from build123d import *

# Parameters (mm, degrees)
SKETCH1_R           = 4
BOSS_EXTRUDE1_DEPTH = 19
SKETCH2_R           = 2.25
CUT_EXTRUDE2_DEPTH  = 19
SKETCH3_R           = 7
SKETCH3_R_2         = 4
BOSS_EXTRUDE2_DEPTH = 3
FILLET1_R           = 1


with BuildPart() as part:
    # Sketch1 → Boss-Extrude1 (new body)
    with BuildSketch(Plane.XY):
        with BuildLine():
            Line((-28.2, 0), (28.2, 0))
            Line((28.2, 0), (28.2, 6))
            Line((28.2, 6), (11.5, 6))
            ThreePointArc((11.5, 6), (10.085786438, 6.585786438), (9.5, 8))
            Line((9.5, 8), (9.5, 11.1))
            ThreePointArc((9.5, 11.1), (0, 20.6), (-9.5, 11.1))
            Line((-9.5, 11.1), (-9.5, 8))
            ThreePointArc((-9.5, 8), (-10.085786438, 6.585786438), (-11.5, 6))
            Line((-11.5, 6), (-28.2, 6))
            Line((-28.2, 6), (-28.2, 0))
        make_face()
        with Locations((0, 11.1)):
            Circle(SKETCH1_R, mode=Mode.SUBTRACT)
    extrude(amount=BOSS_EXTRUDE1_DEPTH)

    # Sketch2 → Cut-Extrude2 (cut)
    with BuildSketch(Plane.XZ):
        with BuildLine():
            Line((28.2, 19), (18.7, 19))
            ThreePointArc((18.7, 19), (25.417514421, 16.217514421), (28.2, 9.5))
            Line((28.2, 9.5), (28.2, 19))
        make_face()
        with BuildLine():
            ThreePointArc((-28.2, 9.5), (-25.417514421, 16.217514421), (-18.7, 19))
            Line((-18.7, 19), (-28.2, 19))
            Line((-28.2, 19), (-28.2, 9.5))
        make_face()
        with BuildLine():
            Line((28.2, 0), (28.2, 9.5))
            ThreePointArc((28.2, 9.5), (25.417514421, 2.782485579), (18.7, 0))
            Line((18.7, 0), (28.2, 0))
        make_face()
        with BuildLine():
            ThreePointArc((-18.7, 0), (-25.417514421, 2.782485579), (-28.2, 9.5))
            Line((-28.2, 9.5), (-28.2, 0))
            Line((-28.2, 0), (-18.7, 0))
        make_face()
        with Locations(Location((19, 9.5, 0), (0, 0, 270))):
            Circle(SKETCH2_R)
        with Locations(Location((-19, 9.5, 0), (0, 0, 270))):
            Circle(SKETCH2_R)
    extrude(amount=-CUT_EXTRUDE2_DEPTH, mode=Mode.SUBTRACT)

    # Sketch3 → Boss-Extrude2 (add)
    with BuildSketch(Plane.XY.offset(19)):
        with Locations((0, 11.1)):
            Circle(SKETCH3_R)
        with Locations((0, 11.1)):
            Circle(SKETCH3_R_2, mode=Mode.SUBTRACT)
    extrude(amount=BOSS_EXTRUDE2_DEPTH)

    # Fillet1
    fillet1_edges = [part.edges().sort_by_distance(p)[0] for p in [
        (10.085786438, 6.585786438, 19),
        (-15.1, 6, 0),
        (-10.085786438, 6.585786438, 0),
        (-9.5, 9.55, 0),
        (0, 20.6, 0),
        (9.5, 9.55, 0),
        (10.085786438, 6.585786438, 0),
        (9.5, 9.55, 19),
        (0, 20.6, 19),
        (-9.5, 9.55, 19),
        (-10.085786438, 6.585786438, 19),
        (-15.1, 6, 19),
        (0, 0, 19),
        (-28.2, 6, 9.5),
        (-28.2, 0, 9.5),
        (0, 0, 0),
        (15.1, 6, 19),
        (28.2, 0, 9.5),
        (28.2, 6, 9.5),
        (15.1, 6, 0),
    ]]
    fillet(fillet1_edges, radius=FILLET1_R)


solid = part.part
Design review of the part built by this model. Coordinates are the model's own, in mm. A direction names the side the tool comes from. Coordinates: 2 decimals unless noted, no trailing zeros. Loops run counter-clockwise (first coordinate to the right, second up) from the corner with the lowest first, then second, coordinate; pieces in that order, holes last.
Item 1: Add section B-B (x = -12.5). Write out the cut boundary in (y, z), and give its area (3 significant figures).
Completed:
outline: (0, 1) arc R1 ccw to (1, 0) - (5, 0) arc R1 ccw to (6, 1) - (6, 18) arc R1 ccw to (5, 19) - (1, 19) arc R1 ccw to (0, 18) - close
area: 113 mm2
Item 2: Draft analysis for pull direction Z (two halves, no side actions). For faces 6 (the cylindrical face through (16.804, 2.958, 9.988)), 7 (the cylindrical face through (-21.196, 2.958, 9.988)), 8 (the flat face through (0, 0, 9)), 9 (the cylindrical face through (15.05, 5.715, 18.699)), state which applies: pulls with the +Z half, pulls with the -Z half, needs draft (parallel to the pull), parting line crosses it, or undercut.
Completed:
face 6: undercut
face 7: undercut
face 8: needs draft
face 9: pulls with the +Z half
Item 3: Add section C-C (x = 17.5). Write out the cut boundary in (y, z), and give its area (3 significant figures).
Completed:
outline: (0, 1) arc R1 ccw to (1, 0) - (5, 0) arc R1 ccw to (6, 1) - (6, 7.82) - (0, 7.82) - close; (0, 11.18) - (6, 11.18) - (6, 18) arc R1 ccw to (5, 19) - (1, 19) arc R1 ccw to (0, 18) - close
area: 93.0 mm2
Item 4: Clearance check with flat-ended pins moving along their axes: pin 1 (6 mm diameter, centred on x = 12, y = 7, fed in from +Z); pin 2 (5 mm diameter, centred on x = -5.5, y = 15.5, fed in from +Z); pin 3 (8 mm diameter, centred on x = -20.5, z = 14.5, fed in from +Y); pin 4 (1.5 mm diameter, centred on y = 10, z = 7, fed in from +X). State where each tip first meets the part, or that it passes through.
Completed:
pin 1: stops at z = 19
pin 2: stops at z = 22
pin 3: stops at y = 6
pin 4: stops at x = 9.5
Item 5: For faces 1 (the cylindrical face through (-9.215, 9.528, 18.699)), 2 (the flat face through (9.5, 10, 9)), 3 (the cylindrical face through (-9.215, 9.572, 0.301)), 4 (the cylindrical face through (3.23, 4.89, 20.48)), 5 (the cylindrical face through (9.215, 9.572, 18.699)), list the 3-axis set-ups (+Z, -Z, +X, -X, +Y, -Y) from which the entire face can be reached by the end or side of a thin tool; tool diameter is ignored.
Completed:
face 1: +Z, -X, +Y
face 2: +Z, -Z, +X, +Y
face 3: -Z, -X, +Y
face 4: +Z
face 5: +Z, +X, +Y
Item 6: Add section A-A (y = 1.75). Write out the cut boundary in (x, z), and give its area (3 significant figures).
Completed:
outline: (-18.7, 0) - (18.7, 0) arc R9.5 ccw to (18.7, 19) - (-18.7, 19) arc R9.5 ccw to start; hole circle Ø4.5 at (-19, 9.5); hole circle Ø4.5 at (19, 9.5)
area: 962 mm2
Item 7: Wall thickness on L1, parallel to X at y = 2.65, z = 9.5; L2, parallel to X at y = 3, z = 11.5; L3, parallel to Y at x = 0, z = 11: over which ranges is each line inside the solid? List them lowest first.
Completed:
L1: x = -28.2 to -21.25, -16.75 to 16.75, 21.25 to 28.2
L2: x = -27.99 to -20.03, -17.97 to 17.97, 20.03 to 27.99
L3: y = 0 to 7.1, 15.1 to 20.6
